Input: part model. Units: mm. Frame: model coordinates. A direction names the side the tool comes from. Coordinates: 2 decimals unless noted, no trailing zeros. Order: outer loops, then holes, each group sorted by start corner. A loop starts at its lowest first (then second) coordinate and runs counter-clockwise, first axis right, second up. Notation, with made-up numbers: M 82.5,-6 L 86.5,-6 A20 ccw 86.5,23 Z; hole C 64.25,87 d3. An arc over 180 degrees is marked long. Answer in a Markdown table with one row per item.
from build123d import *

# Parameters (mm, degrees)
SKETCH1_W           = 88
SKETCH1_H           = 88
BOSS_EXTRUDE1_DEPTH = 3.5
SKETCH2_W           = 86
SKETCH2_H           = 86
CUT_EXTRUDE1_DEPTH  = 2.5
SKETCH3_W           = 52
SKETCH3_H           = 52
CUT_EXTRUDE2_DEPTH  = 2


with BuildPart() as part:
    # Sketch1 → Boss-Extrude1 (new body)
    with BuildSketch(Plane(origin=(0, 0, 0), x_dir=(1, 0, 0), z_dir=(0, 1, 0))):
        Rectangle(SKETCH1_W, SKETCH1_H)
    extrude(amount=BOSS_EXTRUDE1_DEPTH)

    # Sketch2 → Cut-Extrude1 (cut)
    with BuildSketch(Plane(origin=(0, 3.5, 0), x_dir=(1, 0, 0), z_dir=(0, 1, 0))):
        Rectangle(SKETCH2_W, SKETCH2_H)
    extrude(amount=-CUT_EXTRUDE1_DEPTH, mode=Mode.SUBTRACT)

    # Sketch3 → Cut-Extrude2 (cut, through all)
    with BuildSketch(Plane(origin=(0, 1, 0), x_dir=(1, 0, 0), z_dir=(0, 1, 0))):
        Rectangle(SKETCH3_W, SKETCH3_H)
    extrude(amount=-CUT_EXTRUDE2_DEPTH, mode=Mode.SUBTRACT)


solid = part.part
1) Cut plane C-C, the plane y = 2.3. Output: boundary loops of the cut face in (x, z), and give its area (3 significant figures).
Resolved:
| item | result |
|---|---|
| outline | M -44,-44 L 44,-44 L 44,44 L -44,44 Z; hole M -43,-43 L 43,-43 L 43,43 L -43,43 Z |
| area | 348 mm2 |
2) Cut plane D-D, the plane z = 35.5. Output: boundary loops of the cut face in (x, y), and give its area (3 significant figures).
Resolved:
| item | result |
|---|---|
| outline | M -44,0 L 44,0 L 44,3.5 L 43,3.5 L 43,1 L -43,1 L -43,3.5 L -44,3.5 Z |
| area | 93.0 mm2 |
3) Mould query, pull axis X, two halves, no side actions, for faces 1 (the face through (-30, 0, -1)), 2 (the face through (-1, 2, -43)), 3 (the face through (44, 2, 1)). Classes: +X half, -X half, draft (parallel to the pull), parting line (faces both ways), or undercut.
Resolved:
| item | result |
|---|---|
| face 1 | draft |
| face 2 | undercut |
| face 3 | +X half |
4) Reachability of faces 4 (the face through (-1, 2, 43)), 5 (the face through (-1, 2, -44)) from +Z, -Z, +X, -X, +Y, -Y: full face, straight path, thin tool, end or side. Return the list, or none.
Resolved:
| item | result |
|---|---|
| face 4 | +Y |
| face 5 | -Z, +X, -X, +Y, -Y |
5) Cut plane A-A, the plane x = 8.5. Output: boundary loops of the cut face in (y, z).
Resolved:
| item | result |
|---|---|
| outline | M 0,-44 L 3.5,-44 L 3.5,-43 L 1,-43 L 1,-26 L 0,-26 Z; M 0,26 L 1,26 L 1,43 L 3.5,43 L 3.5,44 L 0,44 Z |
6) Cut plane B-B, the plane z = 16. Output: boundary loops of the cut face in (x, y), and give its area (3 significant figures).
Resolved:
| item | result |
|---|---|
| outline | M -44,0 L -26,0 L -26,1 L -43,1 L -43,3.5 L -44,3.5 Z; M 26,0 L 44,0 L 44,3.5 L 43,3.5 L 43,1 L 26,1 Z |
| area | 41.0 mm2 |
7) Material intervals for probe 1 along X at (y, z) = (1.6, -15); probe 2 along X at (y, z) = (0.85, -16), sorted ascending.
Resolved:
| item | result |
|---|---|
| probe 1 | x = -44 to -43, 43 to 44 |
| probe 2 | x = -44 to -26, 26 to 44 |
8) Contact query for a flat-ended pin moving along its axis: pin 1 (12 mm diameter, centred on x = -31.5, z = -20.5, fed in from +Y). Output: stop coordinate, or through.
Resolved:
| item | result |
|---|---|
| pin 1 | stops at y = 1 |
